Geometry: final body of the model. Coordinates: model frame, mm. Face numbers are marked on the shaded views. A direction names the side the tool comes from. Coordinates: 2 decimals unless noted, no trailing zeros. Loops run counter-clockwise (first coordinate to the right, second up) from the corner with the lowest first, then second, coordinate; pieces in that order, holes last. Notation, with made-up numbers: (66, 2.25) - (80, 2.25) arc R29 cw to (80, 26.25) - close; hole circle Ø2 at (71, -6.5). An arc over 180 degrees is marked (long way). Return JSON: item names as keys, results as strings.
from build123d import *

# Parameters (mm, degrees)
TAP_DRILL_FOR_M3X0_5_TAP1_D = 2.5


with BuildPart() as part:
    # Sketch2 → Revolve1 (revolve)
    with BuildSketch(Plane.XY, mode=Mode.PRIVATE) as revolve1_sk:
        Polygon((0, 2.5), (2.5, 2.5), (2.5, 4.5), (4.5, 4.5), (4.5, 2.5), (10, 2.5), (10, 0), (0, 0), align=None)
    revolve(revolve1_sk.sketch.rotate(Axis((0, 0, 0), (0, 1, 0)), 90), axis=Axis((0, 0, 0), (0, 1, 0)))

    # Tap Drill for M3x0.5 Tap1 (through all)
    with Locations(Plane(origin=(0, 2.5, 0), x_dir=(1, 0, 0), z_dir=(0, 1, 0))):
        with Locations((0, 7), (0, -7), (-7, 0), (7, 0), (0, 0)):
            Hole(TAP_DRILL_FOR_M3X0_5_TAP1_D / 2)


solid = part.part
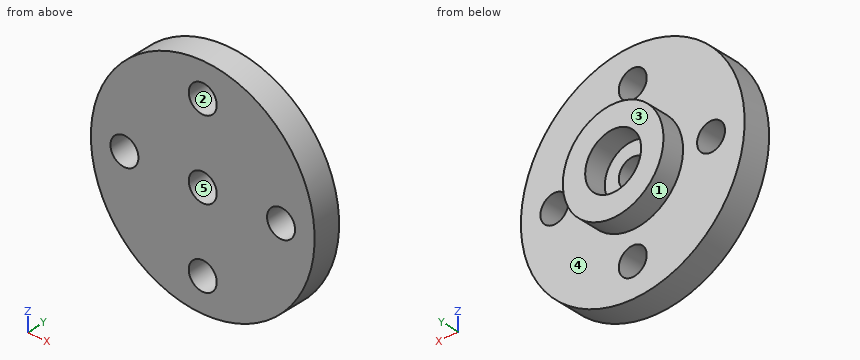
Item 1: Section query C-C, the plane y = 2.2. Return loops of the section in (x, z), and give its area (3 significant figures).
Worked out:
{"outline": "circle Ø20 at (0, 0); hole circle Ø2.5 at (-7, 0); hole circle Ø2.5 at (0, -7); hole circle Ø2.5 at (0, 0); hole circle Ø2.5 at (0, 7); hole circle Ø2.5 at (7, 0)", "area": "290 mm^2"}
Item 2: First-contact query: pin 1 Ø3 at (x, z) = (-5, -2) entering from -Y; pin 2 Ø2 at (x, z) = (-7, 0) entering from +Y; pin 3 Ø3 at (x, z) = (0, 7) entering from +Y; pin 4 Ø1.5 at (x, y) = (-3.5, 3.5) entering from +Z. Flat tips, straight axial feed; report the tip coordinate or a pass-through.
Worked out:
{"pin 1": "y = 0", "pin 2": "through", "pin 3": "y = 2.5", "pin 4": "z = 3.56"}
Item 3: Reachability of the marked faces 4 and 5 from +Z, -Z, +X, -X, +Y, -Y: full face, straight path, thin tool, end or side. Return the list, or none.
Worked out:
{"face 4": "+Y", "face 5": "+Y, -Y"}
Item 4: Mould query, pull axis Z, two halves, no side actions, for the marked faces 1, 2 and 3. Classes: +Z half, -Z half, draft (parallel to the pull), parting line (faces both ways), or undercut.
Worked out:
{"face 1": "parting line", "face 2": "undercut", "face 3": "draft"}
Item 5: Ray query, probe 1 along Y at (x, z) = (1, 9); probe 2 along X at (y, z) = (1.6, 0.75); probe 3 along Z at (x, y) = (-0.5, 1.8). Return the intervals inside material, ascending. Write a range as from..to.
Worked out:
{"probe 1": "0..2.5", "probe 2": "-9.97..-8, -6..-1, 1..6, 8..9.97", "probe 3": "-9.99..-8.15, -5.85..-1.15, 1.15..5.85, 8.15..9.99"}
Item 6: Section query D-D, the plane x = -6.75. Return loops of the section in (y, z).
Worked out:
{"outline": "(0, -7.38) - (2.5, -7.38) - (2.5, -1.22) - (0, -1.22) - close; (0, 1.22) - (2.5, 1.22) - (2.5, 7.38) - (0, 7.38) - close"}
Item 7: Section query A-A, the plane x = 0. Return loops of the section in (y, z).
Worked out:
{"outline": "(0, -10) - (2.5, -10) - (2.5, -8.25) - (0, -8.25) - close; (0, -5.75) - (2.5, -5.75) - (2.5, -4.5) - (4.5, -4.5) - (4.5, -2.5) - (2.5, -2.5) - (2.5, -1.25) - (0, -1.25) - close; (0, 1.25) - (2.5, 1.25) - (2.5, 2.5) - (4.5, 2.5) - (4.5, 4.5) - (2.5, 4.5) - (2.5, 5.75) - (0, 5.75) - close; (0, 8.25) - (2.5, 8.25) - (2.5, 10) - (0, 10) - close"}
Item 8: Section query B-B, the plane z = 0. Return loops of the section in (x, y).
Worked out:
{"outline": "(-10, 0) - (-8.25, 0) - (-8.25, 2.5) - (-10, 2.5) - close; (-5.75, 0) - (-1.25, 0) - (-1.25, 2.5) - (-2.5, 2.5) - (-2.5, 4.5) - (-4.5, 4.5) - (-4.5, 2.5) - (-5.75, 2.5) - close; (1.25, 0) - (5.75, 0) - (5.75, 2.5) - (4.5, 2.5) - (4.5, 4.5) - (2.5, 4.5) - (2.5, 2.5) - (1.25, 2.5) - close; (8.25, 0) - (10, 0) - (10, 2.5) - (8.25, 2.5) - close"}
